Verification items for the finished model (mm, model axes). Round coordinates to 2 decimals unless told otherwise and drop trailing zeros. Write each loop counter-clockwise with the first axis right and the second up, starting at its lowest first coordinate (ties: lowest second). Pieces come first, ordered by that corner, then holes. Notation, with made-up numbers: (-18.5, -19.75) - (25.5, -19.75) arc R34 cw to (25.5, 14.25) - close; hole circle Ø10 at (-36, -33). An arc over 180 degrees is marked (long way). Answer as a JSON object with one key per item and string values. Group by question number.
1) Thickness scan on line 1 (Y direction, x = 3, z = 0.4); line 2 (X direction, y = 107.5, z = 0.45); line 3 (X direction, y = 111.5, z = 0.2). Record the ranges inside material, lowest first.
2) Section check A-A (x = 42). Enter the section's corners in (y, z), then the cut area to 3 significant figures.
3) Go/stop test with a flat-tipped pin: pin 1 Ø2.5 at (x, y) = (289, 28) entering from +Z. Record where the tip stops, or that it passes through.
4) Section check B-B (y = 87). Enter the section's corners in (x, z).
5) Section check C-C (z = 0.3). State how many separate pieces and enclosed holes the cut face has, then the cut area to 3 significant figures.
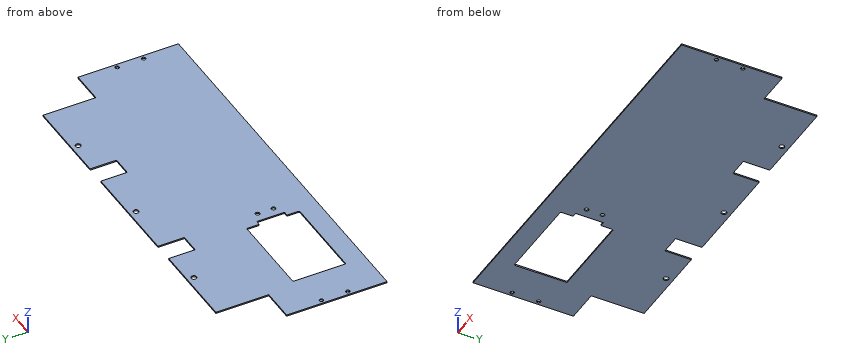
```python
from build123d import *

# Parameters (mm, degrees)
SKETCH_1_R          = 1.5
EXTRUDE_1_DEPTH     = 1
SKETCH_2_R          = 2
SKETCH_2_W          = 15
SKETCH_2_H          = 20
CUT_EXTRUDE_1_DEPTH = 315.198981539
SKETCH_3_W          = 65
SKETCH_3_H          = 40
CUT_EXTRUDE_5_DEPTH = 10
SKETCH_4_W          = 3.5
SKETCH_4_H          = 21
CUT_EXTRUDE_6_DEPTH = 10
SKETCH_6_R          = 1.6
CUT_EXTRUDE_8_DEPTH = 2
FILLET_1_R          = 1


with BuildPart() as part:
    # 草图1 → 凸台-拉伸1 (new body)
    with BuildSketch(Plane.XY):
        Polygon((0, 0), (0, 76), (25, 76), (25, 116), (267, 116), (267, 76), (292, 76), (292, 0), align=None)
        with Locations((3, 48)):
            Circle(SKETCH_1_R, mode=Mode.SUBTRACT)
        with Locations((3, 28)):
            Circle(SKETCH_1_R, mode=Mode.SUBTRACT)
        with Locations(Location((289, 28, 0), (0, 0, 180))):
            Circle(SKETCH_1_R, mode=Mode.SUBTRACT)
        with Locations(Location((289, 48, 0), (0, 0, 180))):
            Circle(SKETCH_1_R, mode=Mode.SUBTRACT)
    extrude(amount=EXTRUDE_1_DEPTH)

    # 草图2 → 切除-拉伸1 (cut, through all)
    with BuildSketch(Plane.XY.offset(1)):
        with Locations((65, 111)):
            Circle(SKETCH_2_R)
        with Locations(Location((227, 111, 0), (0, 0, 180))):
            Circle(SKETCH_2_R)
        with Locations((146, 111)):
            Circle(SKETCH_2_R)
        with Locations((193.5, 106)):
            Rectangle(SKETCH_2_W, SKETCH_2_H)
        with Locations((98.5, 106)):
            Rectangle(SKETCH_2_W, SKETCH_2_H)
    extrude(amount=-CUT_EXTRUDE_1_DEPTH, mode=Mode.SUBTRACT)

    # 草图3 → 切除-拉伸5 (cut)
    with BuildSketch(Plane(origin=(0, 0, 0), x_dir=(-1, 0, 0), z_dir=(0, 0, -1))):
        with Locations((-62.330283152, 34.979584943)):
            Rectangle(SKETCH_3_W, SKETCH_3_H)
    extrude(amount=-CUT_EXTRUDE_5_DEPTH, mode=Mode.SUBTRACT)

    # 草图4 → 切除-拉伸6 (cut)
    with BuildSketch(Plane(origin=(0, 0, 0), x_dir=(-1, 0, 0), z_dir=(0, 0, -1))):
        with Locations((-96.580283152, 34.979584943)):
            Rectangle(SKETCH_4_W, SKETCH_4_H)
    extrude(amount=-CUT_EXTRUDE_6_DEPTH, mode=Mode.SUBTRACT)

    # 草图6 → 切除-拉伸8 (cut)
    with BuildSketch(Plane(origin=(0, 0, 0), x_dir=(-1, 0, 0), z_dir=(0, 0, -1))):
        with Locations((-105.467130331, 28.979584943)):
            Circle(SKETCH_6_R)
        with Locations((-105.467130331, 40.979584943)):
            Circle(SKETCH_6_R)
    extrude(amount=-CUT_EXTRUDE_8_DEPTH, mode=Mode.SUBTRACT)

    # 圆角1
    fillet_1_edges = [part.edges().sort_by_distance(p)[0] for p in [
        (29.830283152, 54.979584943, 0.5),
        (29.830283152, 14.979584943, 0.5),
        (94.830283152, 14.979584943, 0.5),
        (94.830283152, 54.979584943, 0.5),
    ]]
    fillet(fillet_1_edges, radius=FILLET_1_R)


solid = part.part
```
Returned:
{
 "1": {"line 1": "0 to 26.5, 29.5 to 46.5, 49.5 to 76", "line 2": "25 to 91, 106 to 186, 201 to 267", "line 3": "25 to 63.06, 66.94 to 91, 106 to 144.06, 147.94 to 186, 201 to 225.06, 228.94 to 267"},
 "2": {"outline": "(0, 0) - (14.98, 0) - (14.98, 1) - (0, 1) - close; (54.98, 0) - (116, 0) - (116, 1) - (54.98, 1) - close", "area": "76.0 mm2"},
 "3": {"pin 1": "through"},
 "4": {"outline": "(25, 0) - (267, 0) - (267, 1) - (25, 1) - close"},
 "5": {"separate pieces": "1", "enclosed holes": "10", "area": "28,500 mm2"}
}
